Part model, mm, in its own coordinate system. Face numbers are marked on the shaded views. A direction names the side the tool comes from. Round coordinates to 2 decimals unless told otherwise and drop trailing zeros. Order: outer loops, then holes, each group sorted by start corner. A loop starts at its lowest first (then second) coordinate and runs counter-clockwise, first axis right, second up. Notation, with made-up numbers: (-22, 8) - (13, 8) arc R21 ccw to (13, 15) - close; hole circle Ø7 at (78.25, 16.5). An arc over 180 degrees is marked (long way). Answer as a JSON object with one key per item and string values.
```python
from build123d import *

# Parameters (mm, degrees)
F0_W      = 14
F0_H      = 4
F1_DEPTH  = 25
F2_W      = 4
F2_H      = 14
F3_DEPTH  = 10.50036
F4_W      = 14
F4_H      = 4
F5_DEPTH  = 15.21079
F6_W      = 4
F6_H      = 14
F7_DEPTH  = 10.50036
F8_W      = 14
F8_H      = 4
F9_DEPTH  = 11.159998
F10_W     = 4
F10_H     = 14
F11_DEPTH = 8.346948
F12_W     = 14
F12_H     = 4
F13_DEPTH = 30
F15_DEPTH = 3.9999999999
F17_DEPTH = 2
F18_R     = 0.1
F19_R     = 0.25


with BuildPart() as f1:
    # F0 (on Right) → F1 (new body)
    with BuildSketch(Plane.YZ):
        Rectangle(F0_W, F0_H)
    extrude(amount=F1_DEPTH)

    # F2 (on face) → F3 (join)
    with BuildSketch(Plane.XY.offset(2)):
        with Locations((23, 0)):
            Rectangle(F2_W, F2_H)
    extrude(amount=F3_DEPTH)

    # F4 (on face) → F5 (join)
    with BuildSketch(Plane.YZ.offset(25)):
        with Locations((0, 10.50036)):
            Rectangle(F4_W, F4_H)
    extrude(amount=F5_DEPTH)

    # F6 (on face) → F7 (join, through all)
    with BuildSketch(Plane(origin=(0, 0, 8.50036), x_dir=(1, 0, 0), z_dir=(0, 0, -1))):
        with Locations((38.21079, 0)):
            Rectangle(F6_W, F6_H)
    extrude(amount=F7_DEPTH)

    # F8 (on face) → F9 (join)
    with BuildSketch(Plane.YZ.offset(40.21079)):
        Rectangle(F8_W, F8_H)
    extrude(amount=F9_DEPTH)

    # F10 (on face) → F11 (join)
    with BuildSketch(Plane(origin=(0, 0, -2), x_dir=(1, 0, 0), z_dir=(0, 0, -1))):
        with Locations((49.370788, 0)):
            Rectangle(F10_W, F10_H)
    extrude(amount=F11_DEPTH)

    # F12 (on face) → F13 (join)
    with BuildSketch(Plane.YZ.offset(51.370788)):
        with Locations((0, -8.3469480001)):
            Rectangle(F12_W, F12_H)
    extrude(amount=F13_DEPTH)

    # F14 (on face) → F15 (cut, through all)
    with BuildSketch(Plane.XY.offset(-6.3469480001)):
        with BuildLine():
            ThreePointArc((56.370788, -2.0625), (57.8291957362, -1.4584077362), (58.433288, 0))
            ThreePointArc((58.433288, 0), (57.8291957362, 1.4584077362), (56.370788, 2.0625))
            ThreePointArc((56.370788, 2.0625), (54.308288, 0), (56.370788, -2.0625))
        make_face()
        with BuildLine():
            ThreePointArc((56.370788, 2.0625), (57.8291957362, 1.4584077362), (58.433288, 0))
            ThreePointArc((58.433288, 0), (57.8291957362, -1.4584077362), (56.370788, -2.0625))
            Line((56.370788, -2.0625), (75.370788, -2.0625))
            ThreePointArc((75.370788, -2.0625), (73.308288, 0), (75.370788, 2.0625))
            Line((75.370788, 2.0625), (56.370788, 2.0625))
        make_face()
        with BuildLine():
            ThreePointArc((77.433288, 0), (76.8291957362, 1.4584077362), (75.370788, 2.0625))
            ThreePointArc((75.370788, 2.0625), (73.308288, 0), (75.370788, -2.0625))
            ThreePointArc((75.370788, -2.0625), (76.8291957362, -1.4584077362), (77.433288, 0))
        make_face()
    extrude(amount=-F15_DEPTH, mode=Mode.SUBTRACT)

    # F16 (on face) → F17 (cut)
    with BuildSketch(Plane.XY.offset(-6.3469480001)):
        with BuildLine():
            ThreePointArc((56.370788, -4), (59.1992151247, -2.8284271247), (60.370788, 0))
            ThreePointArc((60.370788, 0), (59.1992151247, 2.8284271247), (56.370788, 4))
            ThreePointArc((56.370788, 4), (52.370788, 0), (56.370788, -4))
        make_face()
        with BuildLine():
            ThreePointArc((56.370788, 4), (59.1992151247, 2.8284271247), (60.370788, 0))
            ThreePointArc((60.370788, 0), (59.1992151247, -2.8284271247), (56.370788, -4))
            Line((56.370788, -4), (75.370788, -4))
            ThreePointArc((75.370788, -4), (71.370788, 0), (75.370788, 4))
            Line((75.370788, 4), (56.370788, 4))
        make_face()
        with BuildLine():
            ThreePointArc((79.370788, 0), (78.1992151247, 2.8284271247), (75.370788, 4))
            ThreePointArc((75.370788, 4), (71.370788, 0), (75.370788, -4))
            ThreePointArc((75.370788, -4), (78.1992151247, -2.8284271247), (79.370788, 0))
        make_face()
    extrude(amount=-F17_DEPTH, mode=Mode.SUBTRACT)

    # F18
    f18_edges = [f1.edges().sort_by_distance(p)[0] for p in [
        (52.370788, 0, -6.346948),
        (65.870788, 4, -6.346948),
        (79.370788, 0, -6.346948),
        (65.870788, -4, -6.346948),
        (65.870788, 4, -8.346948),
        (52.370788, 0, -8.346948),
        (54.308288, 0, -8.346948),
        (65.870788, 2.0625, -8.346948),
        (77.433288, 0, -8.346948),
        (79.370788, 0, -8.346948),
        (65.870788, -4, -8.346948),
        (65.870788, -2.0625, -8.346948),
    ]]
    fillet(f18_edges, radius=F18_R)

    # F19
    f19_edges = [f1.edges().sort_by_distance(p)[0] for p in [
        (51.370788, 0, -6.346948),
        (51.370788, 0, 2),
        (40.21079, 0, 2),
        (40.21079, 0, 12.50036),
        (21, 0, 2),
        (21, 0, 12.50036),
        (0, 0, 2),
        (0, 0, -2),
        (25, 0, -2),
        (25, 0, 8.50036),
        (36.21079, 0, 8.50036),
        (47.370788, 0, -2),
        (47.370788, 0, -10.346948),
        (81.370788, 0, -10.346948),
        (81.370788, 0, -6.346948),
        (36.21079, 0, -2),
    ]]
    fillet(f19_edges, radius=F19_R)


solid = f1.part
```
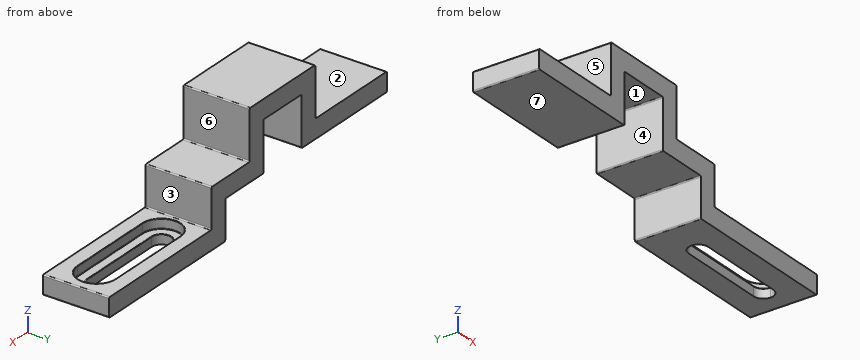
Item 1: Drop flat-ended pins along their axis: P1, Ø4, axis at x = 13.5, y = -0.5, coming from the -Z side; P2, Ø8, axis at x = 58, z = -5.5, coming from the -Y side; P3, Ø4, axis at y = -3, z = -0.5, coming from the +X side; P4, Ø5, axis at y = 3, z = 5, coming from the -X side. Give the stop position or say it passes through.
Taken from the geometry:
{"P1": "z = -2", "P2": "y = -7", "P3": "x = 51.37", "P4": "x = 21"}
Item 2: Two-plate mould, pull along X, no slides. Class the marked faces 1, 2 and 3: pulls with the +X half, pulls with the -X half, needs draft (parallel to the pull), parting line crosses it, or undercut.
Taken from the geometry:
{"face 1": "undercut", "face 2": "needs draft", "face 3": "pulls with the +X half"}
Item 3: Probe L1, parallel to X at y = 2, z = 4; L2, parallel to X at y = -4, z = -1; L3, parallel to X at y = 2.25, z = -2.75. List the from-to ranges inside material, lowest first. Write a range as from..to.
Taken from the geometry:
{"L1": "21..25, 36.21..40.21", "L2": "0..25, 36.21..51.37", "L3": "47.37..51.37"}
Item 4: Cut at D-D (z = 5). Write the cut outline in (x, y).
Taken from the geometry:
{"outline": "(21, -7) - (25, -7) - (25, 7) - (21, 7) - close; (36.21, -7) - (40.21, -7) - (40.21, 7) - (36.21, 7) - close"}
Item 5: Cut at A-A (x = 62.5). Write the cut outline in (y, z).
Taken from the geometry:
{"outline": "(-7, -10.35) - (-2.06, -10.35) - (-2.06, -8.45) arc R0.1 ccw to (-2.16, -8.35) - (-3.9, -8.35) arc R0.1 cw to (-4, -8.25) - (-4, -6.45) arc R0.1 ccw to (-4.1, -6.35) - (-7, -6.35) - close; (2.06, -10.35) - (7, -10.35) - (7, -6.35) - (4.1, -6.35) arc R0.1 ccw to (4, -6.45) - (4, -8.25) arc R0.1 cw to (3.9, -8.35) - (2.16, -8.35) arc R0.1 ccw to (2.06, -8.45) - close"}
Item 6: Cut at B-B (z = 0). Write the cut outline in (x, y).
Taken from the geometry:
{"outline": "(0, -7) - (25, -7) - (25, 7) - (0, 7) - close; (36.21, -7) - (51.37, -7) - (51.37, 7) - (36.21, 7) - close"}
Item 7: Tool access for the marked faces 4, 5, 6 and 7: list every direction of +Z, -Z, +X, -X, +Y, -Y with a clear straight run to the whole face (end or side of a thin tool).
Taken from the geometry:
{"face 4": "-Z, +Y, -Y", "face 5": "+Z, -X, +Y, -Y", "face 6": "+Z, +X, +Y, -Y", "face 7": "-Z, -X, +Y, -Y"}
